Check sheet for the modelled part. Datum: model origin and axes. Units: mm. Round coordinates to 2 decimals unless told otherwise and drop trailing zeros. Write each loop counter-clockwise with the first axis right and the second up, starting at its lowest first coordinate (ties: lowest second). Pieces come first, ordered by that corner, then holes. Notation, with made-up numbers: (-24.75, -17.5) - (13.25, -17.5) arc R36 ccw to (13.25, 19.5) - close; hole circle Ø9 at (49.25, -23.75). An arc over 180 degrees is marked (long way). Answer as a JSON object with one key per item and string values. Group by question number.
Item 1: Sectioned sample at B-B on x = 1.25. Record the boundary of the cut face in (y, z).
Item 2: Gauge pin test, flat ends, axial feed: P1, Ø3, axis at x = 6.5, z = 4.5, coming from the -Y side; P2, Ø7, axis at x = -0.25, y = 90, coming from the -Z side; P3, Ø4, axis at y = 68, z = 5, coming from the +X side; P4, Ø1, axis at y = 15, z = -2, coming from the +X side. Record the tip position at first contact, or that the pin passes through.
Item 3: Thickness scan on line 1 (Y direction, x = 0, z = 3) (3 decimals); line 2 (Y direction, x = -2, z = 8.75); line 3 (X direction, y = 87.5, z = 1). Record the ranges inside material, lowest first.
Item 4: Sectioned sample at C-C on y = 43.5. Record the boundary of the cut face in (x, z), plus the area to 3 significant figures.
Item 5: Release check for a two-part mould opening along X. For faces 1 (the cylindrical face through (0.275, -12.497, 0.14)), 2 (the cylindrical face through (1.59, 86.45, 0.14)), 3 (the flat face through (0, 45, 10)) record: pulls with the +X half, pulls with the -X half, needs draft (parallel to the pull), parting line crosses it, or undercut.
Item 6: Sectioned sample at A-A on z = 8.75. Record the boundary of the cut face in (x, y) (3 decimals), plus the area to 3 significant figures.
```python
from build123d import *

# Parameters (mm, degrees)
EXTRUDE1_DEPTH     = 10
SKETCH6_R          = 4
CUT_EXTRUDE1_DEPTH = 21
SKETCH8_R          = 6.975
CUT_EXTRUDE2_DEPTH = 21


with BuildPart() as part:
    # Sketch2 → Extrude1 (new body, symmetric)
    with BuildSketch(Plane.XY):
        with BuildLine():
            Line((-12.5, 0), (-10, 92.232909937))
            ThreePointArc((-10, 92.232909937), (0.871187265, 99.936304296), (9.747437125, 89.999645621))
            Line((9.747437125, 89.999645621), (12.5, 0))
            ThreePointArc((12.5, 0), (0, -12.5), (-12.5, 0))
        make_face()
    extrude(amount=EXTRUDE1_DEPTH, both=True)

    # Sketch6 → Cut-Extrude1 (cut, through all)
    with BuildSketch(Plane.XY.offset(10)):
        with Locations((-0.252562875, 89.999645621)):
            Circle(SKETCH6_R)
    extrude(amount=-CUT_EXTRUDE1_DEPTH, mode=Mode.SUBTRACT)

    # Sketch8 → Cut-Extrude2 (cut, through all)
    with BuildSketch(Plane.XY.offset(10)):
        Circle(SKETCH8_R)
    extrude(amount=-CUT_EXTRUDE2_DEPTH, mode=Mode.SUBTRACT)


solid = part.part
```
Completed:
{
 "1": {"outline": "(-12.44, -10) - (-6.86, -10) - (-6.86, 10) - (-12.44, 10) - close; (6.86, -10) - (86.29, -10) - (86.29, 10) - (6.86, 10) - close; (93.71, -10) - (99.89, -10) - (99.89, 10) - (93.71, 10) - close"},
 "2": {"P1": "y = -11.46", "P2": "through", "P3": "x = 10.48", "P4": "x = 12.06"},
 "3": {"line 1": "-12.5 to -6.975, 6.975 to 86.008, 93.992 to 99.996", "line 2": "-12.34 to -6.68, 6.68 to 86.4, 93.6 to 99.85", "line 3": "-10.13 to -3.38, 2.87 to 9.82"},
 "4": {"outline": "(-11.32, -10) - (11.17, -10) - (11.17, 10) - (-11.32, 10) - close", "area": "450 mm²"},
 "5": {"face 1": "parting line crosses it", "face 2": "undercut", "face 3": "needs draft"},
 "6": {"outline": "(-12.5, 0) arc R12.5 ccw to (12.5, 0) - (9.747, 90) arc R10 ccw to (-10, 92.233) - close; hole circle Ø13.95 at (0, 0); hole circle Ø8 at (-0.253, 90)", "area": "2,220 mm²"}
}
